Input: part model. Units: mm. Frame: model coordinates. A direction names the side the tool comes from. Round coordinates to 2 decimals unless told otherwise and drop trailing zeros. Loops run counter-clockwise (first coordinate to the right, second up) from the corner with the lowest first, then second, coordinate; pieces in that order, holes last. Notation, with made-up numbers: (6.25, -8) - (16.25, -8) arc R13 cw to (16.25, -4) - close; hole circle Ø7 at (17, 46). An arc over 180 degrees is marked (long way). One line per question, with ' | ' between items. Start each with the question number.
from build123d import *

# Parameters (mm, degrees)
CROQUIS1_W              = 170
CROQUIS1_H              = 140
SALIENTE_EXTRUIR1_DEPTH = 30
CHAFL_N1_SIZE           = 5
CROQUIS2_R              = 20
SALIENTE_EXTRUIR2_DEPTH = 30
CROQUIS2_3_R            = 5
CORTAR_EXTRUIR1_DEPTH   = 30


with BuildPart() as part:
    # Croquis1 → Saliente-Extruir1 (new body)
    with BuildSketch(Plane.XY):
        Rectangle(CROQUIS1_W, CROQUIS1_H)
    extrude(amount=SALIENTE_EXTRUIR1_DEPTH)

    # Chaflán1
    chafl_n1_edges = [part.edges().sort_by_distance(p)[0] for p in [
        (85, -70, 15),
        (-85, -70, 15),
        (-85, 70, 15),
        (85, 70, 15),
    ]]
    chamfer(chafl_n1_edges, length=CHAFL_N1_SIZE)

    # Croquis2 → Saliente-Extruir2 (add)
    with BuildSketch(Plane.XY.offset(30)):
        with Locations((15, 0)):
            Circle(CROQUIS2_R)
    extrude(amount=SALIENTE_EXTRUIR2_DEPTH)

    # Croquis2<3> → Cortar-Extruir1 (cut)
    with BuildSketch(Plane.XY.offset(30)):
        with Locations((-75, 60)):
            Circle(CROQUIS2_3_R)
        with Locations((-75, -60)):
            Circle(CROQUIS2_3_R)
    extrude(amount=-CORTAR_EXTRUIR1_DEPTH, mode=Mode.SUBTRACT)


solid = part.part
(1) Line query: line 1 along Y through (x, z) = (-75, 19); line 2 along Z through (x, y) = (15, -61.5); line 3 along X through (y, z) = (3, 42.5). Output: solid intervals per line, ascending. Write a range as from..to.
(2) Section B-B, the plane y = 60. Output: boundary loops of the cut face in (x, z), plus the area to 3 significant figures.
(3) Reachability of faces 1 (the face through (82, 68, 15)), 2 (the face through (-4.98, 0.88, 44.79)) from +Z, -Z, +X, -X, +Y, -Y: full face, straight path, thin tool, end or side. Return the list, or none.
(4) Section A-A, the plane x = -75. Output: boundary loops of the cut face in (y, z), plus the area to 3 significant figures.
(5) Section D-D, the plane x = 15. Output: boundary loops of the cut face in (y, z).
(6) Pin query (flat end, axial travel): P1, Ø10, axis at x = 44, y = -35.5, coming from the +Z side; P2, Ø6, axis at x = 25, z = 33.5, coming from the -Y side (3 decimals). Return the tip coordinate at first contact, or that it passes through.
(7) Pull-direction query (X, two-part tool) for faces 3 (the face through (83, -67, 15)), 4 (the face through (15, 0, 60)), 5 (the face through (-72, 64, 15)); classes: released by +X, released by -X, zero draft, split by the parting line, or undercut.
(8) Section C-C, the plane y = 0. Output: boundary loops of the cut face in (x, z), plus the area to 3 significant figures.
Derived:
1) line 1: y = -70..-65, -55..55, 65..70 | line 2: z = 0..30 | line 3: x = -4.77..34.77
2) outline: (-85, 0) - (-80, 0) - (-80, 30) - (-85, 30) - close; (-70, 0) - (85, 0) - (85, 30) - (-70, 30) - close | area: 4,800 mm²
3) face 1: +Z, -Z, +X, +Y | face 2: +Z
4) outline: (-70, 0) - (-65, 0) - (-65, 30) - (-70, 30) - close; (-55, 0) - (55, 0) - (55, 30) - (-55, 30) - close; (65, 0) - (70, 0) - (70, 30) - (65, 30) - close | area: 3,600 mm²
5) outline: (-70, 0) - (70, 0) - (70, 30) - (20, 30) - (20, 60) - (-20, 60) - (-20, 30) - (-70, 30) - close
6) P1: stops at z = 30 | P2: stops at y = -18.735
7) face 3: released by +X | face 4: zero draft | face 5: undercut
8) outline: (-85, 0) - (85, 0) - (85, 30) - (35, 30) - (35, 60) - (-5, 60) - (-5, 30) - (-85, 30) - close | area: 6,300 mm²
